from build123d import *

# Parameters (mm, degrees)
F0_W         = 65
F0_H         = 35
F1_DEPTH     = 15
F2_R         = 17.825
F3_DEPTH     = 15
F4_W         = 39
F4_H         = 37.65
F5_DEPTH     = 8.06
F7_DEPTH     = 15.001
F8_W         = 30.8607626557
F8_H         = 37.5567990541
F9_DEPTH     = 1
F10_W        = 25.4967134297
F10_H        = 35
F11_DEPTH    = 1
F12_SIZE     = 2
F13_R        = 2.75
F14_DEPTH    = 6.941
F15_R        = 10.44
F16_DEPTH    = 1.5
F17_R        = 4.5
F19_DEPTH    = 25
F20_W        = 7
F20_H        = 3
F20_W_2      = 3
F20_H_2      = 7
F21_DEPTH    = 1.7
F22_T1_DEPTH = 15.7437221591
F22_T3_DEPTH = 15.7437221591
F22_T5_DEPTH = 11.3718610795
F22_T7_DEPTH = 15.7437221591
F3_FACE1_R   = 2.75
F23_DEPTH    = 3
F23_TAPER    = 30


# Not quite as in the source:
# - a fillet or chamfer that OpenCascade refuses, or shapes differently, is made with other operations: its cross-section is extruded or revolved along the edge and cut away or added


with BuildPart() as f1:
    # F0 (on Front) → F1 (new body)
    with BuildSketch(Plane.XZ):
        Rectangle(F0_W, F0_H)
    extrude(amount=F1_DEPTH)

    # F2 (on face) → F3 (join, through all)
    with BuildSketch(Plane.XZ.offset(15)):
        with Locations((15.675, 0)):
            Circle(F2_R)
    extrude(amount=-F3_DEPTH)

    # F4 (on face) → F5 (cut)
    with BuildSketch(Plane.XZ.offset(15)):
        with Locations((15, 0)):
            Rectangle(F4_W, F4_H)
    extrude(amount=-F5_DEPTH, mode=Mode.SUBTRACT)

    # F6 (on face) → F7 (cut, through all)
    with BuildSketch(Plane.XZ.offset(15)):
        Polygon((-9, 16.23), (-9, 17.5), (-32.5, 17.5), (-32.5, 15.93), align=None)
        Polygon((-32.5, -17.5), (-9, -17.5), (-9, -16.23), (-32.5, -15.93), align=None)
    extrude(amount=-F7_DEPTH, mode=Mode.SUBTRACT)

    # F8 (on face) → F9 (cut)
    with BuildSketch(Plane.XZ.offset(15)):
        with Locations((-24.4303813279, 1.2783995271)):
            Rectangle(F8_W, F8_H)
    extrude(amount=-F9_DEPTH, mode=Mode.SUBTRACT)

    # F10 (on face) → F11 (cut)
    with BuildSketch(Plane(origin=(0, 0, 0), x_dir=(-1, 0, 0), z_dir=(0, 1, 0))):
        with Locations((21.7483567148, 0)):
            Rectangle(F10_W, F10_H)
    extrude(amount=-F11_DEPTH, mode=Mode.SUBTRACT)

    # F12
    f12_edges = [f1.edges().sort_by_distance(p)[0] for p in [
        (-4.5, -6.94, 0),
    ]]
    chamfer(f12_edges, length=F12_SIZE)

    # F13 (on face) → F14 (cut, through all)
    with BuildSketch(Plane.XZ.offset(6.94)):
        with Locations((15.675, 0)):
            Circle(F13_R)
    extrude(amount=-F14_DEPTH, mode=Mode.SUBTRACT)

    # F15 (on face) → F16 (cut)
    with BuildSketch(Plane.XZ.offset(6.94)):
        with Locations((15.675, 0)):
            Circle(F15_R)
    extrude(amount=-F16_DEPTH, mode=Mode.SUBTRACT)

    # F17
    f17_edges = [f1.edges().sort_by_distance(p)[0] for p in [
        (-20.75, -1, 16.08),
        (-20.75, -1, -16.08),
    ]]
    fillet(f17_edges, radius=F17_R)

    # F18 (on face) → F19 (cut)
    with BuildSketch(Plane.XZ.offset(6.94)):
        with BuildLine():
            ThreePointArc((15.675, 17.825), (33.5, 0), (15.675, -17.825))
            Line((15.675, -17.825), (14.3514294177, -24.9375402927))
            Line((14.3514294177, -24.9375402927), (39.8063696921, -24.9375402927))
            Line((39.8063696921, -24.9375402927), (43.452385813, 22.5534923375))
            Line((43.452385813, 22.5534923375), (15.675, 27.0696729422))
            Line((15.675, 27.0696729422), (15.675, 17.825))
        make_face()
    extrude(amount=-F19_DEPTH, mode=Mode.SUBTRACT)

    # F20 (on face) → F21 (join)
    with BuildSketch(Plane.XZ.offset(6.94)):
        with Locations((30, 0)):
            Rectangle(F20_W, F20_H)
        with Locations((15.675, 14.325)):
            Rectangle(F20_W_2, F20_H_2)
        with Locations((1.35, 0)):
            Rectangle(F20_W, F20_H)
        with Locations((15.675, -14.325)):
            Rectangle(F20_W_2, F20_H_2)
    extrude(amount=F21_DEPTH)

    # F22: chamfer of 1.7 on 8 edges, made by hand

    # F22_s2 → F22_t1 (cut)
    with BuildSketch(Plane.YZ.offset(22.1281389205)):
        Polygon((-6.94, 1.5), (-8.64, -0.2), (-8.64, 1.5), align=None)
        Polygon((-6.94, -1.5), (-8.64, 0.2), (-8.64, -1.5), align=None)
    extrude(amount=F22_T1_DEPTH, mode=Mode.SUBTRACT)

    # F22_s4 → F22_t3 (cut)
    with BuildSketch(Plane.XY.offset(-22.1968610795)):
        Polygon((17.175, -6.94), (15.475, -8.64), (17.175, -8.64), align=None)
        Polygon((14.175, -6.94), (15.875, -8.64), (14.175, -8.64), align=None)
    extrude(amount=F22_T3_DEPTH, mode=Mode.SUBTRACT)

    # F22_s6 → F22_t5 (cut)
    with BuildSketch(Plane.YZ.offset(-2.15)):
        Polygon((-6.94, -1.5), (-8.64, 0.2), (-8.64, -1.5), align=None)
        Polygon((-6.94, 1.5), (-8.64, -0.2), (-8.64, 1.5), align=None)
    extrude(amount=F22_T5_DEPTH, mode=Mode.SUBTRACT)

    # F22_s8 → F22_t7 (cut)
    with BuildSketch(Plane.XY.offset(6.4531389205)):
        Polygon((14.175, -6.94), (15.875, -8.64), (14.175, -8.64), align=None)
        Polygon((17.175, -6.94), (15.475, -8.64), (17.175, -8.64), align=None)
    extrude(amount=F22_T7_DEPTH, mode=Mode.SUBTRACT)

    # F3_face1 (on face) → F23 (join)
    with BuildSketch(Plane(origin=(0.7743209172, 0, 0), x_dir=(-1, 0, 0), z_dir=(0, 1, 0))):
        with BuildLine():
            Line((-11.5123719834, -17.5), (9.7743209172, -17.5))
            Line((9.7743209172, -17.5), (9.7743209172, 17.5))
            Line((9.7743209172, 17.5), (-11.5123719834, 17.5))
            ThreePointArc((-11.5123719834, 17.5), (-32.7256790828, 0), (-11.5123719834, -17.5))
        make_face()
        with Locations((-14.9006790828, 0)):
            Circle(F3_FACE1_R, mode=Mode.SUBTRACT)
    extrude(amount=F23_DEPTH, taper=F23_TAPER)


solid = f1.part
Could you check a few things on this model? Use its own coordinates, in mm. A direction names the side the tool comes from. Coordinates: 2 decimals unless noted, no trailing zeros. Loops run counter-clockwise (first coordinate to the right, second up) from the corner with the lowest first, then second, coordinate; pieces in that order, holes last.
1. Imagine slicing it at A-A (y = -11). Please give me the cut outline in (x, z), and give its area (3 significant figures).
2. For P1, Ø16.5, axis at x = 15, z = 5, coming from the -Y side; P2, Ø7.5, axis at x = 6.5, y = -7.5, coming from the +Z side; P3, Ø1.5, axis at x = -22, y = -13, coming from the +Z side, each with a flat end and sliding along its axis, tell me the tip position at first contact or that it passes through.
3. We'd pull the mould along X, two halves only. Please class faces 5 (the face through (26.5, -8, 0)), 6 (the face through (16.436, -7.68, -14.374)), 7 (the face through (-21, -14, 0)): released by +X, released by -X, zero draft, split by the parting line, or undercut.
4. I need wall thicknesses on L1, parallel to X at y = -1.2, z = 0 (3 decimals); L2, parallel to Y at x = -25, z = -6; L3, parallel to X at y = -10, z = 1.5. Which ranges of each line are inside material? Lowest first, please.
5. For faces 1 (the face through (7.39, -6.2, -6.35)), 2 (the face through (-3.51, -7.95, -0.24)), 3 (the face through (29.95, -7.68, -0.76)), 4 (the face through (-20.597, -2.283, 14.729)), which set-ups out of +Z, -Z, +X, -X, +Y, -Y let a thin tool reach every point of the face, with its end or its side?
Computed values:
1. outline: (-32.5, -15.93) - (-9, -16.23) - (-9, -17.5) - (-4.5, -17.5) - (-4.5, 17.5) - (-9, 17.5) - (-9, 16.23) - (-32.5, 15.93) - close
1. area: 913 mm2
2. P1: stops at y = -8.44
2. P2: stops at z = 17.5
2. P3: stops at z = 16.07
3. face 5: undercut
3. face 6: released by +X
3. face 7: zero draft
4. L1: x = -32.5 to 12.925, 18.425 to 33.5
4. L2: y = -14 to -1
4. L3: x = -32.5 to -4.5
5. face 1: -Y
5. face 2: +Z, -Z, -Y
5. face 3: -Z, +X, -Y
5. face 4: +Z, -X, +Y
